Here's the drawing with two shaded views (mm, measured from the low corner). I have some questions. Coordinates: 2 decimals unless noted, no trailing zeros. Order: outer loops, then holes, each group sorted by start corner. A loop starts at its lowest first (then second) coordinate and runs counter-clockwise, first axis right, second up. Notation, with made-up numbers: (48.25, 38) - (91.25, 38) arc R28 cw to (91.25, 71) - close; hole circle Ø3 at (11, -29). An arc over 180 degrees is marked (long way). One line per item, written item: value. Start each with the question number.
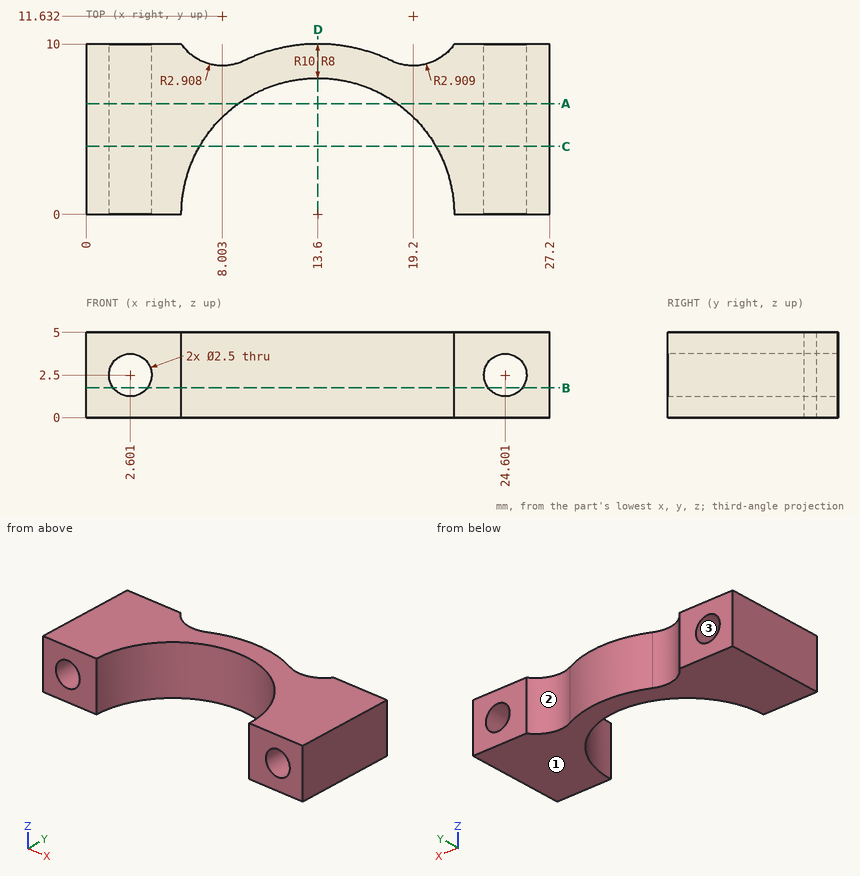
Q1. If I drill on L1, parallel to X at y = 4, z = 3.2 (1 decimal); L2, parallel to X at y = 6.75, z = 1.6 (1 decimal); L3, parallel to Z at x = 2, y = 8 (1 decimal), over which ranges is the centre line in solid material (lowest first)?
Q2. I want a section at B-B on z = 1.75. Please give me the cut outline in (x, y) (1 decimal).
Q3. I'm going to push a flat-ended pin straight in: pin 1 (1 mm diameter, centred on x = 19.5, z = 2, fed in from -Y). Where does the tip first touch, or does it pass through?
Q4. We'd pull the mould along Z, two halves only. Please class the marked faces 1, 2 and 3: +Z half, -Z half, draft (parallel to the pull), parting line (faces both ways), or undercut.
Q5. I want a section at A-A on y = 6.5. Please give me the cut outline in (x, z).
Q6. I want a section at C-C on y = 4. Please give me the cut outline in (x, z).
Q7. I want a section at D-D on x = 13.6. Please give me the cut outline in (y, z).
Values follow:
1. L1: x = 0 to 1.6, 3.6 to 6.7, 20.5 to 23.6, 25.6 to 27.2
1. L2: x = 0 to 1.7, 3.5 to 9.3, 17.9 to 23.7, 25.5 to 27.2
1. L3: z = 0 to 1.4, 3.6 to 5
2. outline: (0, 0) - (1.6, 0) - (1.6, 10) - (0, 10) - close; (3.6, 0) - (5.6, 0) arc R8 cw to (21.6, 0) - (23.6, 0) - (23.6, 10) - (21.6, 10) arc R2.9 cw to (17.9, 9) arc R10 ccw to (9.3, 9) arc R2.9 cw to (5.6, 10) - (3.6, 10) - close; (25.6, 0) - (27.2, 0) - (27.2, 10) - (25.6, 10) - close
3. pin 1: stops at y = 4.8
4. face 1: -Z half
4. face 2: draft
4. face 3: undercut
5. outline: (0, 0) - (8.94, 0) - (8.94, 5) - (0, 5) - close; (18.26, 0) - (27.2, 0) - (27.2, 5) - (18.26, 5) - close; hole circle Ø2.5 at (2.6, 2.5); hole circle Ø2.5 at (24.6, 2.5)
6. outline: (0, 0) - (6.67, 0) - (6.67, 5) - (0, 5) - close; (20.53, 0) - (27.2, 0) - (27.2, 5) - (20.53, 5) - close; hole circle Ø2.5 at (2.6, 2.5); hole circle Ø2.5 at (24.6, 2.5)
7. outline: (8, 0) - (10, 0) - (10, 5) - (8, 5) - close
